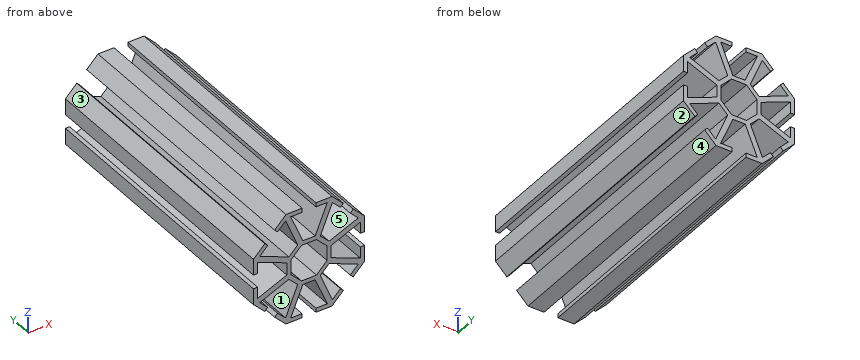
from build123d import *

# Parameters (mm, degrees)
F1_DEPTH        = 100
F3_DEPTH        = 100.001
F3_COPIES_COUNT = 8
F4_W            = 5
F4_H            = 1.5
F5_DEPTH        = 100.001
F5_COPIES_COUNT = 8


# Not quite as in the source:
# - a pattern or mirror of a feature is missing from the dataset's text; its kind, count and spacing are read off the source's solid


with BuildPart() as f1:
    # F0 (on Front) → F1 (new body)
    with BuildSketch(Plane.XZ):
        Polygon((8.2842712475, 20), (-8.2842712475, 20), (-20, 8.2842712475), (-20, -8.2842712475), (-8.2842712475, -20), (8.2842712475, -20), (20, -8.2842712475), (20, 8.2842712475), align=None)
        Polygon((-6.5, 2.6923881554), (-2.6923881554, 6.5), (2.6923881554, 6.5), (6.5, 2.6923881554), (6.5, -2.6923881554), (2.6923881554, -6.5), (-2.6923881554, -6.5), (-6.5, -2.6923881554), align=None, mode=Mode.SUBTRACT)
    extrude(amount=F1_DEPTH)

    # F2 (on face) → F3 (cut, through all)
    with BuildSketch(Plane.XZ.offset(100)):
        Polygon((-6.5805587036, 18.5), (-2.2313162987, 8), (2.2313162987, 8), (6.5805587036, 18.5), align=None)
    f3 = extrude(amount=-F3_DEPTH, mode=Mode.SUBTRACT)

    # F3_copies: F3 ×8 about axis
    f3_copies_axis = Axis((0, 0, 0), (0, 1, 0))
    for i in range(1, F3_COPIES_COUNT):
        add(f3.rotate(f3_copies_axis, i * 360 / F3_COPIES_COUNT), mode=Mode.SUBTRACT)

    # F4 (on face) → F5 (cut, through all)
    with BuildSketch(Plane.XZ.offset(100)):
        with Locations((0, 19.25)):
            Rectangle(F4_W, F4_H)
    f5 = extrude(amount=-F5_DEPTH, mode=Mode.SUBTRACT)

    # F5_copies: F5 ×8 about axis
    f5_copies_axis = Axis((0, 0, 0), (0, 1, 0))
    for i in range(1, F5_COPIES_COUNT):
        add(f5.rotate(f5_copies_axis, i * 360 / F5_COPIES_COUNT), mode=Mode.SUBTRACT)


solid = f1.part
Verification items for the finished model (mm, model axes). Face numbers are marked on the shaded views. A direction names the side the tool comes from. Give positions to 0.01 mm unless a question says otherwise; leave off trailing zeros. Write each loop counter-clockwise with the first axis right and the second up, starting at its lowest first coordinate (ties: lowest second). Pieces come first, ordered by that corner, then holes. Notation, with made-up numbers: M 60,59.5 L 111,59.5 A30 ccw 111,82.5 Z; hole C -32,3 d10. An arc over 180 degrees is marked long. Write item = value, one per line.
(1) Go/stop test with flat-tipped pins: pin 1 Ø2 at (x, y) = (1, -39.5) entering from +Z; pin 2 Ø2 at (y, z) = (-67, 0) entering from +X; pin 3 Ø1.5 at (y, z) = (-20.5, 10.5) entering from -X; pin 4 Ø3 at (x, z) = (12.5, 10) entering from -Y. Record where each tip stops, or that it passes through.
Found:
pin_1 = 8
pin_2 = 8
pin_3 = -18.53
pin_4 = through
(2) Sectioned sample at A-A (x = -10). Record the cut outline in (y, z), then the cut area to 3 significant figures.
Found:
outline = M -100,-18.28 L 0,-18.28 L 0,-16.16 L -100,-16.16 Z; M -100,-5.22 L 0,-5.22 L 0,-3.06 L -100,-3.06 Z; M -100,3.06 L 0,3.06 L 0,5.22 L -100,5.22 Z; M -100,16.16 L 0,16.16 L 0,18.28 L -100,18.28 Z
area = 857 mm2
(3) Access from +Z, -Z, +X, -X, +Y, -Y to the whole of each face (thin tool, end or side, straight path). Record for the marked faces 4 and 5.
Found:
face_4 = -Z, +X, +Y, -Y
face_5 = +Y, -Y
(4) Draft check along Z on the marked faces 1, 2 and 3. Enter one of: released by +Z, released by -Z, zero draft, split by the parting line, or undercut.
Found:
face_1 = undercut
face_2 = released by -Z
face_3 = released by +Z
(5) Material ranges on line 1 (Z direction, x = -11, y = -34.5); line 2 (Z direction, x = 16, y = -45); line 3 (X direction, y = -66.5, z = 1.5), recorded low to high.
Found:
line_1 = -17.28 to -15.16, -5.64 to -3.47, 3.47 to 5.64, 15.16 to 17.28
line_2 = -12.28 to -10.16, -7.71 to -5.55, 5.55 to 7.71, 10.16 to 12.28
line_3 = -8 to -6.5, 6.5 to 8
